from build123d import *

# Parameters (mm, degrees)
SKETCH1_W           = 80
SKETCH1_H           = 40
BOSS_EXTRUDE1_DEPTH = 20
SKETCH2_W           = 10.2
SKETCH2_H           = 20
CUT_EXTRUDE1_DEPTH  = 81
SKETCH3_R           = 4.125
CUT_EXTRUDE2_DEPTH  = 21
CHAMFER1_SIZE       = 0.5
CHAMFER1_SIZE2      = 0.866025404


with BuildPart() as part:
    # Sketch1 → Boss-Extrude1 (new body)
    with BuildSketch(Plane(origin=(0, 0, 0), x_dir=(1, 0, 0), z_dir=(0, 1, 0))):
        Rectangle(SKETCH1_W, SKETCH1_H)
    extrude(amount=BOSS_EXTRUDE1_DEPTH)

    # Sketch2 → Cut-Extrude1 (cut, through all)
    with BuildSketch(Plane.ZY.offset(40)):
        Rectangle(SKETCH2_W, SKETCH2_H)
    extrude(amount=-CUT_EXTRUDE1_DEPTH, mode=Mode.SUBTRACT)

    # Sketch3 → Cut-Extrude2 (cut, through all)
    with BuildSketch(Plane(origin=(0, 20, 0), x_dir=(1, 0, 0), z_dir=(0, 1, 0))):
        with Locations(Location((12.5, -11.5, 0), (0, 0, 270))):  # turned: the seam where the file's is
            Circle(SKETCH3_R)
        with Locations(Location((-12.5, -11.5, 0), (0, 0, 270))):  # turned: the seam where the file's is
            Circle(SKETCH3_R)
        with Locations(Location((-12.5, 11.5, 0), (0, 0, 270))):  # turned: the seam where the file's is
            Circle(SKETCH3_R)
        with Locations(Location((12.5, 11.5, 0), (0, 0, 270))):  # turned: the seam where the file's is
            Circle(SKETCH3_R)
        with Locations(Location((30, -11.5, 0), (0, 0, 270))):  # turned: the seam where the file's is
            Circle(SKETCH3_R)
        with Locations(Location((-30, -11.5, 0), (0, 0, 270))):  # turned: the seam where the file's is
            Circle(SKETCH3_R)
        with Locations(Location((-30, 11.5, 0), (0, 0, 270))):  # turned: the seam where the file's is
            Circle(SKETCH3_R)
        with Locations(Location((30, 11.5, 0), (0, 0, 270))):  # turned: the seam where the file's is
            Circle(SKETCH3_R)
        with Locations(Location((0, 0, 0), (0, 0, 270))):  # turned: the seam where the file's is
            Circle(SKETCH3_R)
    extrude(amount=-CUT_EXTRUDE2_DEPTH, mode=Mode.SUBTRACT)

    # Chamfer1
    chamfer1_edges = [part.edges().sort_by_distance(p)[0] for p in [
        (12.5, 20, 7.375),
        (0, 20, -4.125),
        (30, 20, -15.625),
        (-30, 20, -15.625),
        (-30, 20, 7.375),
        (30, 20, 7.375),
        (12.5, 20, -15.625),
        (-12.5, 20, -15.625),
        (-12.5, 20, 7.375),
    ]]
    chamfer1_side = [part.faces().sort_by_distance(p)[0] for p in [
        (0, 20, 19.105572809),
    ]]
    chamfer(chamfer1_edges, length=CHAMFER1_SIZE, length2=CHAMFER1_SIZE2, reference=chamfer1_side[0])


solid = part.part
Design review of the part built by this model. Coordinates are the model's own, in mm. A direction names the side the tool comes from. Coordinates: 2 decimals unless noted, no trailing zeros. Order: outer loops, then holes, each group sorted by start corner. A loop starts at its lowest first (then second) coordinate and runs counter-clockwise, first axis right, second up. Notation, with made-up numbers: (-39.75, 39.25) -> (-2.75, 39.25) arc R10 ccw to (-2.75, 53.25) -> close; hole circle Ø3 at (38, 67). An arc over 180 degrees is marked (long way). Use one line per item in the form item = value. Start each with the question number.
(1) Add section B-B on z = 0. State the section outline as (x, y) points (3 decimals).
(2) Add section C-C on x = 30. State the section outline as (y, z) points (3 decimals).
(3) Insertion check: pin 1 (5 mm diameter, centred on x = 4.5, z = -1.5, fed in from -Y); pin 2 (10 mm diameter, centred on y = 4, z = 0, fed in from -X). Each pin has a flat end and moves straight along its axis. Give the tip position at first contact, or say it passes through.
(4) For probe 1 along X at (y, z) = (9, 11.5) (3 decimals); probe 2 along Z at (x, y) = (18, 3); probe 3 along Z at (x, y) = (28, 14.5), list the stretches that pass through material, from the lowest coordinate up.
(5) Add section D-D on z = -11.5. State the section outline as (x, y) points (3 decimals), plus the area to 3 significant figures.
(6) For faces 4 (the cylindrical face through (-25.91, 9.7, -12.04)), 5 (the flat face through (-1, 5, 5.1)), list the 3-axis set-ups (+Z, -Z, +X, -X, +Y, -Y) from which the entire face can be reached by the end or side of a thin tool; tool diameter is ignored.
(7) The part is to be moulded in two halves that separate along X. For faces 1 (the cylindrical face through (9.99, 9.701, 8.227)), 2 (the flat face through (40, 12, 0)), 3 (the flat face through (-0.6, 10, -4.6)), say which applies: +X half, -X half, draft (parallel to the pull), parting line (faces both ways), or undercut.
(8) Add section A-A on y = 8.75. Give the number of separate pieces and of enclosed holes in the cut face, plus the area to 3 significant figures.
Answer block:
q1.outline = (-40, 10) -> (-4.125, 10) -> (-4.125, 19.134) -> (-4.625, 20) -> (-40, 20) -> close; (4.125, 10) -> (40, 10) -> (40, 20) -> (4.625, 20) -> (4.125, 19.134) -> close
q2.outline = (0, -20) -> (20, -20) -> (20, -16.125) -> (19.134, -15.625) -> (0, -15.625) -> close; (0, -7.375) -> (19.134, -7.375) -> (20, -6.875) -> (20, 6.875) -> (19.134, 7.375) -> (0, 7.375) -> (0, 5.1) -> (10, 5.1) -> (10, -5.1) -> (0, -5.1) -> close; (0, 15.625) -> (19.134, 15.625) -> (20, 16.125) -> (20, 20) -> (0, 20) -> close
q3.pin_1 = 10
q3.pin_2 = through
q4.probe_1 = -40 to -34.125, -25.875 to -16.625, -8.375 to 8.375, 16.625 to 25.875, 34.125 to 40
q4.probe_2 = -20 to -5.1, 5.1 to 20
q4.probe_3 = -20 to -15.11, -7.89 to 7.89, 15.11 to 20
q5.outline = (-40, 0) -> (-34.125, 0) -> (-34.125, 19.134) -> (-34.625, 20) -> (-40, 20) -> close; (-25.875, 0) -> (-16.625, 0) -> (-16.625, 19.134) -> (-17.125, 20) -> (-25.375, 20) -> (-25.875, 19.134) -> close; (-8.375, 0) -> (8.375, 0) -> (8.375, 19.134) -> (7.875, 20) -> (-7.875, 20) -> (-8.375, 19.134) -> close; (16.625, 0) -> (25.875, 0) -> (25.875, 19.134) -> (25.375, 20) -> (17.125, 20) -> (16.625, 19.134) -> close; (34.125, 0) -> (40, 0) -> (40, 20) -> (34.625, 20) -> (34.125, 19.134) -> close
q5.area = 938 mm²
q6.face_4 = +Y, -Y
q6.face_5 = +X, -X, -Y
q7.face_1 = undercut
q7.face_2 = +X half
q7.face_3 = draft
q8.separate_pieces = 2
q8.enclosed_holes = 8
q8.area = 1,960 mm²
